from build123d import *

# Parameters (mm, degrees)
SKETCH1_R           = 1.575
BOSS_EXTRUDE1_DEPTH = 9.525
SKETCH2_W           = 3.205
SKETCH2_H           = 10
CUT_EXTRUDE4_DEPTH  = 9.525
SKETCH4_R           = 1.4224
CUT_EXTRUDE5_DEPTH  = 3
SKETCH5_R           = 3.2385
CUT_EXTRUDE6_DEPTH  = 2.2
CUT_EXTRUDE6_TAPER  = 55


with BuildPart() as part:
    # Sketch1 → Boss-Extrude1 (new body)
    with BuildSketch(Plane.XY):
        with BuildLine():
            Line((4.7625, 10.5), (4.7625, 3))
            Line((4.7625, 3), (12.5, 3))
            Line((12.5, 3), (12.5, 0))
            Line((12.5, 0), (-12.5, 0))
            Line((-12.5, 0), (-12.5, 3))
            Line((-12.5, 3), (-4.7625, 3))
            Line((-4.7625, 3), (-4.7625, 10.5))
            ThreePointArc((-4.7625, 10.5), (0, 15.2625), (4.7625, 10.5))
        make_face()
        with Locations((0, 10.5)):
            Circle(SKETCH1_R, mode=Mode.SUBTRACT)
    extrude(amount=BOSS_EXTRUDE1_DEPTH)

    # Sketch2 → Cut-Extrude4 (cut)
    with BuildSketch(Plane.ZY.offset(4.7625)):
        with Locations((4.7625, 10.2625)):
            Rectangle(SKETCH2_W, SKETCH2_H)
    extrude(amount=-CUT_EXTRUDE4_DEPTH, mode=Mode.SUBTRACT)

    # Sketch4 → Cut-Extrude5 (cut)
    with BuildSketch(Plane(origin=(0, 3, 0), x_dir=(1, 0, 0), z_dir=(0, 1, 0))):
        with Locations((8.63125, -4.7625)):
            Circle(SKETCH4_R)
        with Locations((-8.63125, -4.7625)):
            Circle(SKETCH4_R)
    extrude(amount=-CUT_EXTRUDE5_DEPTH, mode=Mode.SUBTRACT)

    # Sketch5 → Cut-Extrude6 (cut)
    with BuildSketch(Plane(origin=(0, 3, 0), x_dir=(1, 0, 0), z_dir=(0, 1, 0))):
        with Locations((8.63125, -4.7625)):
            Circle(SKETCH5_R)
        with Locations((-8.63125, -4.7625)):
            Circle(SKETCH5_R)
    extrude(amount=-CUT_EXTRUDE6_DEPTH, taper=CUT_EXTRUDE6_TAPER, mode=Mode.SUBTRACT)


solid = part.part
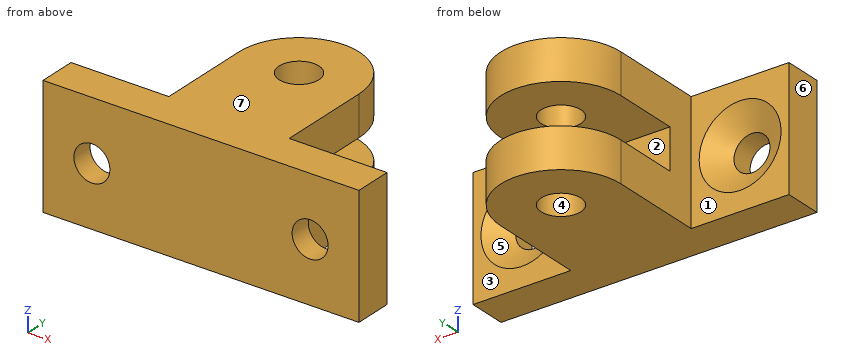
The model under review builds one solid part; all positions refer to its coordinate system, in mm. Face numbers are marked on the shaded views. A direction names the side the tool comes from. Round coordinates to 2 decimals unless told otherwise and drop trailing zeros. Order: outer loops, then holes, each group sorted by start corner. A loop starts at its lowest first (then second) coordinate and runs counter-clockwise, first axis right, second up. Notation, with made-up numbers: (38, 34) -> (64, 34) arc R15 ccw to (64, 56) -> close; hole circle Ø5 at (-34.75, -20.5). An arc over 180 degrees is marked (long way). Use CSV: the item, a comma, the result in double quotes. Start each with the question number.
(1) Consider section C-C on y = 9.5. Write out the cut boundary in (x, z) (1 decimal).
(2) Consider section B-B on x = 0. Write out the cut boundary in (y, z) (1 decimal).
(3) Mouldability with a two-part tool opening along X and no side actions: class the marked faces 5, 6 and 7 as pulls with the +X half, pulls with the -X half, needs draft (parallel to the pull), parting line crosses it, or undercut.
(4) Consider section A-A on y = 6.75. Write out the cut boundary in (x, z) (1 decimal), and give its area (3 significant figures).
(5) Consider section D-D on x = -4.25. Write out the cut boundary in (y, z) (1 decimal), and give its area (3 significant figures).
(6) Insertion check: pin 1 (3 mm diameter, centred on x = -1.5, y = 10.5, fed in from -Z); pin 2 (1 mm diameter, centred on x = -1, z = 4, fed in from +Y); pin 3 (2.5 mm diameter, centred on x = -8.63, z = 4.76, fed in from +Y); pin 4 (4 mm diameter, centred on x = 10, z = 7, fed in from +Y). Each pin has a flat end and moves straight along its axis. Give the tip position at first contact, or say it passes through.
(7) Wall thickness on probe 1 along Y at (x, z) = (0, 1.45) (1 decimal); probe 2 along Z at (x, y) = (2.75, 10.25) (3 decimals); probe 3 along Y at (x, z) = (-7.25, 9): over which ranges is each line inside the solid? List them lowest first. Write a range as from..to.
(8) Tool access review of the marked faces 1, 2, 3 and 4: name each direction out of +Z, -Z, +X, -X, +Y, -Y from which nothing blocks a thin tool from reaching the whole face with its end or side.
Responses:
1,outline,"(-4.8, 0) -> (-1.2, 0) -> (-1.2, 3.2) -> (-4.8, 3.2) -> close; (-4.8, 6.4) -> (-1.2, 6.4) -> (-1.2, 9.5) -> (-4.8, 9.5) -> close; (1.2, 0) -> (4.8, 0) -> (4.8, 3.2) -> (1.2, 3.2) -> close; (1.2, 6.4) -> (4.8, 6.4) -> (4.8, 9.5) -> (1.2, 9.5) -> close"
2,outline,"(0, 0) -> (8.9, 0) -> (8.9, 3.2) -> (5.3, 3.2) -> (5.3, 6.4) -> (8.9, 6.4) -> (8.9, 9.5) -> (0, 9.5) -> close; (12.1, 0) -> (15.3, 0) -> (15.3, 3.2) -> (12.1, 3.2) -> close; (12.1, 6.4) -> (15.3, 6.4) -> (15.3, 9.5) -> (12.1, 9.5) -> close"
3,face 5,"undercut"
3,face 6,"pulls with the -X half"
3,face 7,"needs draft"
4,outline,"(-4.8, 0) -> (4.8, 0) -> (4.8, 3.2) -> (-4.8, 3.2) -> close; (-4.8, 6.4) -> (4.8, 6.4) -> (4.8, 9.5) -> (-4.8, 9.5) -> close"
4,area,"60.2 mm²"
5,outline,"(0, 0) -> (12.6, 0) -> (12.6, 3.2) -> (5.3, 3.2) -> (5.3, 6.4) -> (12.6, 6.4) -> (12.6, 9.5) -> (0, 9.5) -> close"
5,area,"96.8 mm²"
6,pin 1,"z = 0"
6,pin 2,"y = 5.26"
6,pin 3,"through"
6,pin 4,"y = 3"
7,probe 1,"0..8.9, 12.1..15.3"
7,probe 2,"0..3.16, 6.365..9.525"
7,probe 3,"0..3"
8,face 1,"+Z, -Z, -X, +Y"
8,face 2,"+X, -X, +Y"
8,face 3,"+Z, -Z, +X, +Y"
8,face 4,"+Z, -Z"
